Geometry: final body of the model. Coordinates: model frame, mm. A direction names the side the tool comes from. Give positions to 0.01 mm unless a question says otherwise; leave off trailing zeros. Write each loop counter-clockwise with the first axis right and the second up, starting at its lowest first coordinate (ties: lowest second). Pieces come first, ordered by that corner, then holes. Notation, with made-up numbers: (-4, 23.5) - (23, 23.5) arc R27 ccw to (23, 41.5) - close; hole circle Ø11 at (68.25, -19). An arc over 180 degrees is marked (long way). Return JSON: item names as keys, results as strings.
from build123d import *

# Parameters (mm, degrees)
SKETCH1_R           = 62.5
SKETCH1_R_2         = 44.5
BOSS_EXTRUDE1_DEPTH = 6
CUT_EXTRUDE1_START  = 55
SKETCH2_R           = 2
CUT_EXTRUDE1_DEPTH  = 10
CUT_EXTRUDE2_START  = -65
SKETCH2_2_R         = 2
CUT_EXTRUDE2_DEPTH  = 10
CUT_EXTRUDE3_START  = 55
SKETCH3_R           = 2
CUT_EXTRUDE3_DEPTH  = 10
CUT_EXTRUDE4_START  = -65
SKETCH3_2_R         = 2
CUT_EXTRUDE4_DEPTH  = 10


with BuildPart() as part:
    # Sketch1 → Boss-Extrude1 (new, symmetric)
    with BuildSketch(Plane.XY):
        Circle(SKETCH1_R)
        Circle(SKETCH1_R_2, mode=Mode.SUBTRACT)
    extrude(amount=BOSS_EXTRUDE1_DEPTH, both=True)

    # Sketch2 → Cut-Extrude1 (cut)
    with BuildSketch(Plane(origin=(0, 0, 0), x_dir=(1, 0, 0), z_dir=(0, 1, 0)).offset(CUT_EXTRUDE1_START)):
        with Locations(Location((0, 0, 0), (0, 0, 90))):
            Circle(SKETCH2_R)
    extrude(amount=CUT_EXTRUDE1_DEPTH, mode=Mode.SUBTRACT)

    # Sketch2_2 → Cut-Extrude2 (cut)
    with BuildSketch(Plane(origin=(0, 0, 0), x_dir=(1, 0, 0), z_dir=(0, 1, 0)).offset(CUT_EXTRUDE2_START)):
        with Locations(Location((0, 0, 0), (0, 0, 90))):
            Circle(SKETCH2_2_R)
    extrude(amount=CUT_EXTRUDE2_DEPTH, mode=Mode.SUBTRACT)

    # Sketch3 → Cut-Extrude3 (cut)
    with BuildSketch(Plane(origin=(0, 0, 0), x_dir=(0, 0, -1), z_dir=(1, 0, 0)).offset(CUT_EXTRUDE3_START)):
        Circle(SKETCH3_R)
    extrude(amount=CUT_EXTRUDE3_DEPTH, mode=Mode.SUBTRACT)

    # Sketch3_2 → Cut-Extrude4 (cut)
    with BuildSketch(Plane(origin=(0, 0, 0), x_dir=(0, 0, -1), z_dir=(1, 0, 0)).offset(CUT_EXTRUDE4_START)):
        Circle(SKETCH3_2_R)
    extrude(amount=CUT_EXTRUDE4_DEPTH, mode=Mode.SUBTRACT)


solid = part.part
Q1. Pin query (flat end, axial travel): P1, Ø5, axis at y = -43, z = -2, coming from the -X side; P2, Ø5, axis at y = 42, z = 3.5, coming from the -X side; P3, Ø3.5, axis at x = 0, z = 0, coming from the +Y side. Return the tip coordinate at first contact, or that it passes through.
Answer key:
{"P1": "stops at x = -47.6", "P2": "stops at x = -48.44", "P3": "stops at y = 55"}
Q2. Section query C-C, the plane z = 0. Return the cut outline in (x, y), plus the area to 3 significant figures.
Answer key:
{"outline": "(-62.47, -2) arc R62.5 ccw to (-2, -62.47) - (-2, -55) - (2, -55) - (2, -62.47) arc R62.5 ccw to (62.47, -2) - (55, -2) - (55, 2) - (62.47, 2) arc R62.5 ccw to (2, 62.47) - (2, 55) - (-2, 55) - (-2, 62.47) arc R62.5 ccw to (-62.47, 2) - (-55, 2) - (-55, -2) - close; hole circle Ø89 at (0, 0)", "area": "5,930 mm^2"}
Q3. Material intervals for probe 1 along Z at (x, y) = (60, 0); probe 2 along X at (y, z) = (14, -1.75); probe 3 along X at (y, z) = (-18, 2.75), sorted ascending. Write a range as [from, to].
Answer key:
{"probe 1": "z = [-6, -2], [2, 6]", "probe 2": "x = [-60.91, -42.24], [42.24, 60.91]", "probe 3": "x = [-59.85, -40.7], [40.7, 59.85]"}
Q4. Set-up query: faces 1 (the cylindrical face through (2, -59, 0)), 2 (the cylindrical face through (-58.803, -1.774, -0.923)), 3 (the flat face through (0, 55, 0)). Return all of +Z, -Z, +X, -X, +Y, -Y with unobstructed straight access to the full face (end or side cutting, diameter ignored); none if empty.
Answer key:
{"face 1": "-Y", "face 2": "-X", "face 3": "+Y"}
Q5. Section query A-A, the plane y = 0. Return the cut outline in (x, z), plus the area to 3 significant figures.
Answer key:
{"outline": "(-62.5, -6) - (-44.5, -6) - (-44.5, 6) - (-62.5, 6) - (-62.5, 2) - (-55, 2) - (-55, -2) - (-62.5, -2) - close; (44.5, -6) - (62.5, -6) - (62.5, -2) - (55, -2) - (55, 2) - (62.5, 2) - (62.5, 6) - (44.5, 6) - close", "area": "372 mm^2"}
Q6. Mould query, pull axis X, two halves, no side actions, for faces 4 (the cylindrical face through (58.698, -1.774, -0.923)), 5 (the cylindrical face through (2, 59, 0)), 6 (the flat face through (55, 0, 0)). Classes: pulls with the +X half, pulls with the -X half, needs draft (parallel to the pull), parting line crosses it, or undercut.
Answer key:
{"face 4": "needs draft", "face 5": "undercut", "face 6": "pulls with the +X half"}
Q7. Section query D-D, the plane y = 30.5. Return the cut outline in (x, z), plus the area to 3 significant figures.
Answer key:
{"outline": "(-54.55, -6) - (-32.4, -6) - (-32.4, 6) - (-54.55, 6) - close; (32.4, -6) - (54.55, -6) - (54.55, 6) - (32.4, 6) - close", "area": "532 mm^2"}
Q8. Section query B-B, the plane x = -20. Return the cut outline in (y, z).
Answer key:
{"outline": "(-59.21, -6) - (-39.75, -6) - (-39.75, 6) - (-59.21, 6) - close; (39.75, -6) - (59.21, -6) - (59.21, 6) - (39.75, 6) - close"}
